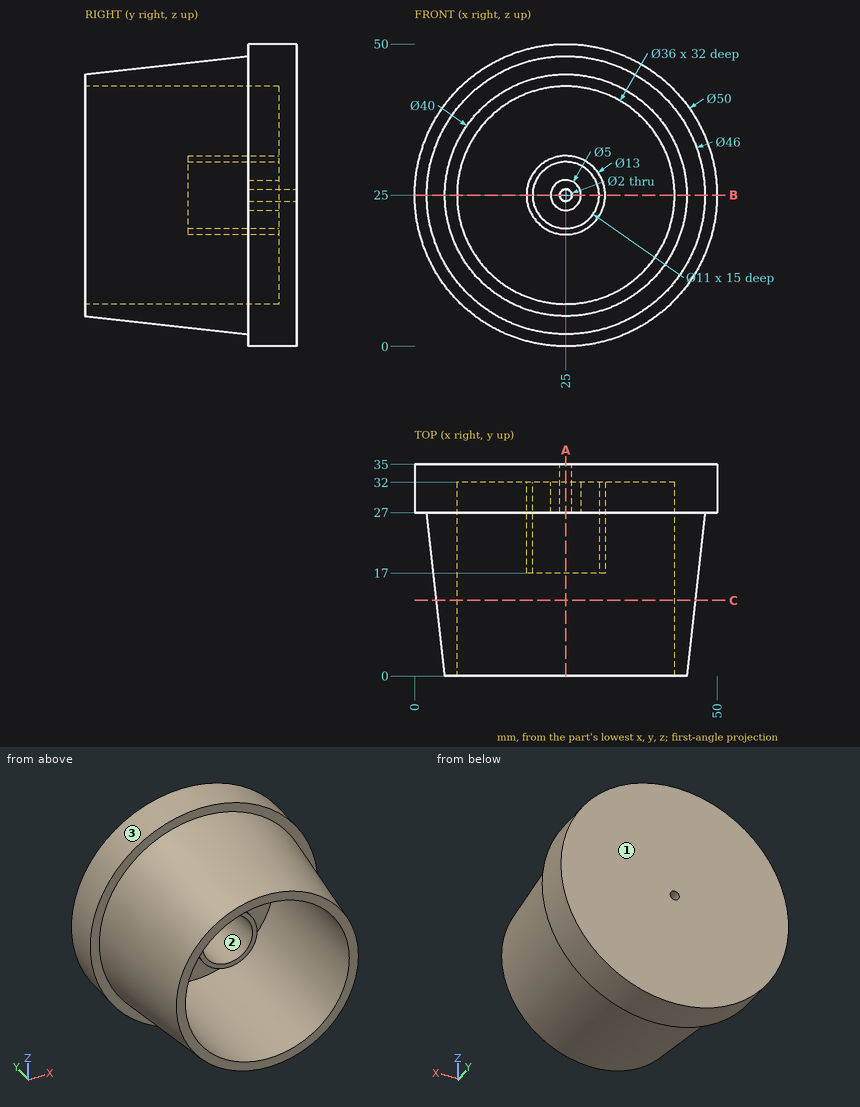
Part print with two shaded views. Sizes in mm from the minimum x, y, z corner. Round coordinates to 2 decimals unless told otherwise and drop trailing zeros. Order: outer loops, then holes, each group sorted by start corner. A loop starts at its lowest first (then second) coordinate and runs counter-clockwise, first axis right, second up.
(1) Pin check, flat tips, straight feed: pin 1 (5 mm diameter, centred on y = 15.5, z = 35, fed in from -X); pin 2 (6.5 mm diameter, centred on x = 24.5, z = 25, fed in from -Y); pin 3 (6 mm diameter, centred on x = 35.5, y = 26.5, fed in from +Z); pin 4 (18 mm diameter, centred on x = 33.5, z = 19, fed in from -Y). Stop position of each tip, or through.
(2) Band-saw the part on A-A (x = 25). List the corners of the cut face in (y, z), then the cut area to 3 significant figures.
(3) Pull direction Z, two halves, no side cores. Call the marked faces 1, 2 and 3: released by +Z, released by -Z, zero draft, split by the parting line, or undercut.
(4) Band-saw the part on B-B (z = 25). List the corners of the cut face in (x, y), then the cut area to 3 significant figures.
(5) Band-saw the part on C-C (y = 12.5). List the corners of the cut face in (x, z).
(6) Drill centre lines: line 1 (Z direction, x = 25, y = 29); line 2 (Z direction, x = 25, y = 33); line 3 (Y direction, x = 33, z = 29). Where is each one in solid material? Low to high.
Verdict:
1. pin 1: stops at x = 4.57
1. pin 2: stops at y = 27
1. pin 3: stops at z = 48.84
1. pin 4: stops at y = 0
2. outline: (0, 5) - (27, 2) - (27, 0) - (35, 0) - (35, 24) - (27, 24) - (27, 22.5) - (32, 22.5) - (32, 19.5) - (17, 19.5) - (17, 18.5) - (32, 18.5) - (32, 7) - (0, 7) - close; (0, 43) - (32, 43) - (32, 31.5) - (17, 31.5) - (17, 30.5) - (32, 30.5) - (32, 27.5) - (27, 27.5) - (27, 26) - (35, 26) - (35, 50) - (27, 50) - (27, 48) - (0, 45) - close
2. area: 448 mm2
3. face 1: zero draft
3. face 2: undercut
3. face 3: split by the parting line
4. outline: (0, 27) - (2, 27) - (5, 0) - (7, 0) - (7, 32) - (18.5, 32) - (18.5, 17) - (19.5, 17) - (19.5, 32) - (22.5, 32) - (22.5, 27) - (24, 27) - (24, 35) - (0, 35) - close; (26, 27) - (27.5, 27) - (27.5, 32) - (30.5, 32) - (30.5, 17) - (31.5, 17) - (31.5, 32) - (43, 32) - (43, 0) - (45, 0) - (48, 27) - (50, 27) - (50, 35) - (26, 35) - close
4. area: 448 mm2
5. outline: circle Ø42.78 at (25, 25); hole circle Ø36 at (25, 25)
6. line 1: z = 0 to 7, 18.5 to 19.5, 22.5 to 24, 26 to 27.5, 30.5 to 31.5, 43 to 50
6. line 2: z = 0 to 24, 26 to 50
6. line 3: y = 32 to 35
